For this review, take the finished solid that the model builds, in its own axes (mm). A direction names the side the tool comes from. Coordinates: 2 decimals unless noted, no trailing zeros. One line per item, written item: value. Start each with the question number.
(1) For faces 4 (the flat face through (0, 22.5, 8)), 5 (the flat face through (-4, -4, -26)), list the 3-axis set-ups (+Z, -Z, +X, -X, +Y, -Y) from which the entire face can be reached by the end or side of a thin tool; tool diameter is ignored.
(2) To check wall thickness, follow line 1 along Z through (x, y) = (-3, -6); line 2 along Y through (x, z) = (-4, 1); line 3 along Y through (x, z) = (2, -19). State the ranges of each line that lie inside material, in increasing order.
(3) Mouldability with a two-part tool opening along Y and no side actions: class faces 1 (the cylindrical face through (4.11, 2.55, -8.05)), 2 (the flat face through (0, -22.5, 8)), 3 (the flat face through (5, 0, 9.4)) as released by +Y, released by -Y, zero draft, split by the parting line, or undercut.
(4) Clearance check with flat-ended pins moving along their axes: pin 1 (2 mm diameter, centred on y = 3.5, z = -13, fed in from +X); pin 2 (4 mm diameter, centred on x = -8, y = 6, fed in from +Z); pin 3 (5 mm diameter, centred on x = -6.5, y = 0.5, fed in from +Z); pin 4 (6 mm diameter, centred on y = 11.5, z = 4, fed in from -X). State where each tip first meets the part, or that it passes through.
```python
from build123d import *

# Parameters (mm, degrees)
SKETCH_4_R          = 8.5
CUT_EXTRUDE_1_DEPTH = 33.4
SKETCH_5_R          = 3
CUT_EXTRUDE_2_DEPTH = 33.4
EXTRUDE_START       = 2
SKETCH_6_W          = 45
SKETCH_6_H          = 45
SKETCH_6_R          = 8.5
EXTRUDE_1_DEPTH     = 2


with BuildPart() as part:
    # 草图1 → 放样1 section 0
    with BuildSketch(Plane.XY):
        with BuildLine():
            Line((-18.25, 18.25), (18.25, 18.25))
            Line((18.25, 18.25), (18.25, -18.25))
            Line((18.25, -18.25), (-18.25, -18.25))
            Line((-18.25, -18.25), (-18.25, 18.25))
        make_face()
    # 草图2 → 放样1 section 1
    with BuildSketch(Plane.XY.offset(7.4)):
        with BuildLine():
            Line((-22.5, 22.5), (22.5, 22.5))
            Line((22.5, 22.5), (22.5, -22.5))
            Line((22.5, -22.5), (-22.5, -22.5))
            Line((-22.5, -22.5), (-22.5, 22.5))
        make_face()
    loft()

    # 草图3 → section 0 of loft_2
    with BuildSketch(Plane(origin=(0, 0, -29), x_dir=(-1, 0, 0), z_dir=(0, 0, -1)), mode=Mode.PRIVATE) as loft_2_s0:
        with BuildLine():
            Line((-15, 15), (15, 15))
            Line((15, 15), (15, -15))
            Line((15, -15), (-15, -15))
            Line((-15, -15), (-15, 15))
        make_face()
    # loft up to a face of the part (loft_2)
    loft([loft_2_s0.sketch, part.faces().sort_by_distance((0, 0, 0))[0]])

    # 草图4 → 切除-拉伸1 (cut)
    with BuildSketch(Plane.XY.offset(7.4)):
        with Locations((-4, 0)):
            Circle(SKETCH_4_R)
    extrude(amount=-CUT_EXTRUDE_1_DEPTH, mode=Mode.SUBTRACT)

    # 草图5 → 切除-拉伸2 (cut)
    with BuildSketch(Plane.XY.offset(-26)):
        with Locations((-4, 0)):
            Circle(SKETCH_5_R)
    extrude(amount=-CUT_EXTRUDE_2_DEPTH, mode=Mode.SUBTRACT)

    # 草图6 → 凸台-拉伸1 (add)
    with BuildSketch(Plane.XY.offset(7.4).offset(EXTRUDE_START)):
        Rectangle(SKETCH_6_W, SKETCH_6_H)
        with Locations((-4, 0)):
            Circle(SKETCH_6_R, mode=Mode.SUBTRACT)
    extrude(amount=-EXTRUDE_1_DEPTH)


solid = part.part
```
Geometry check:
1. face 4: +Z, -Z, +X, -X, +Y
1. face 5: +Z
2. line 1: z = -29 to -26
2. line 2: y = -18.82 to -8.5, 8.5 to 18.82
2. line 3: y = -16.12 to -6.02, 6.02 to 16.12
3. face 1: undercut
3. face 2: released by -Y
3. face 3: zero draft
4. pin 1: stops at x = 16.91
4. pin 2: stops at z = 9.4
4. pin 3: stops at z = -26
4. pin 4: stops at x = -22.27
